Input: part model. Units: mm. Frame: model coordinates. A direction names the side the tool comes from. Round coordinates to 2 decimals unless told otherwise and drop trailing zeros. Write each loop counter-clockwise with the first axis right and the second up, starting at its lowest first coordinate (ties: lowest second). Pieces come first, ordered by that corner, then holes. Notation, with made-up numbers: (-22, 40.25) - (-9, 40.25) arc R18 ccw to (-9, 66.25) - close; hole circle Ø11 at (18.5, -10.75). An arc over 180 degrees is marked (long way). One line per item, written item: value. Start each with the question number.
Autodesk Inventor part; units mm, degrees
ref_plane "YZ Plane" through (0, 0, 0) normal (1, 0, 0) x (0, 1, 0)
ref_plane "XZ Plane" through (0, 0, 0) normal (0, 1, 0) x (-1, 0, 0)
ref_plane "XY Plane" through (0, 0, 0) normal (0, 0, 1) x (1, 0, 0)
sketch "Sketch1" plane through (0, 0, 0) normal (0, 0, 1) x (1, 0, 0)
  circle A0 centre (0, 0) radius 15
  dimension "d0" = 30
extrude "Extrusion1" add sketch "Sketch1" along normal blind 19
sketch "Sketch2" plane through (0, 0, 19) normal (0, 0, 1) x (1, 0, 0)
  circle A0 centre (0, 0) radius 3
  dimension "d3" = 6
extrude "Extrusion2" cut sketch "Sketch2" against normal blind 19
sketch "Sketch3" plane through (0, 0, 0) normal (0, 0, -1) x (-1, 0, 0)
  circle A0 centre (0, 0) radius 15
extrude "Extrusion3" add sketch "Sketch3" along normal blind 5
sketch "Sketch6" plane through (0, 0, -5) normal (0, 0, -1) x (-1, 0, 0)
  line L0 (0, -8) -> (-6.9282, -4)
  line L1 (-6.9282, -4) -> (-6.9282, 4)
  line L2 (-6.9282, 4) -> (0, 8)
  line L3 (0, 8) -> (6.9282, 4)
  line L4 (6.9282, 4) -> (6.9282, -4)
  line L5 (6.9282, -4) -> (0, -8)
  point P0 (0, 0)
  point P1 (0, 0)
  dimension "d15" = 16
extrude "Extrusion6" cut sketch "Sketch6" against normal blind 5
sketch "Sketch7" plane through (0, 0, 0) normal (1, 0, 0) x (0, 1, 0)
  circle A0 centre (0, 10) radius 1.4
  point P0 (0, 0)
  dimension "d18" = 2.8
  dimension "d19" = 10
extrude "Extrusion7" cut sketch "Sketch7" along normal through all
properties part number "FA012" material "ABS Plastic"
Q1. Pull-direction query (Y, two-part tool) for faces 3 (the flat face through (-3.1, -6.5, -5)), 4 (the cylindrical face through (8.74, -0.303, 11.367)), 5 (the flat face through (-3.416, 6.028, -2.535)); classes: pulls with the +Y half, pulls with the -Y half, needs draft (parallel to the pull), parting line crosses it, or undercut.
Q2. Cut plane B-B, the plane y = 0. Output: boundary loops of the cut face in (x, z), and give its area (3 significant figures).
Q3. Contact query for flat-ended pins moving along their axis: pin 1 Ø1.5 at (y, z) = (-10.5, 0.5) entering from +X; pin 2 Ø1.5 at (y, z) = (2, -2.5) entering from -X; pin 3 Ø1.5 at (x, z) = (9, 7.5) entering from -Y; pin 4 Ø3.5 at (x, y) = (0, 0) entering from -Z. Output: stop coordinate, or through.
Q4. Material intervals for probe 1 along Y at (x, z) = (0, 11.75); probe 2 along X at (y, z) = (6, -2.25); probe 3 along Y at (x, z) = (7.25, 10), sorted ascending. Write a range as from..to.
Q5. Cut plane C-C, the plane x = 0.5. Output: boundary loops of the cut face in (y, z), and give its area (3 significant figures).
Q6. Access query for faces 1 (the cylindrical face through (-3, 0, 10)), 2 (the flat face through (-3.513, -5.972, -2.535)). Directions: +Z, -Z, +X, -X, +Y, -Y. A direction counts if a zero-diameter tool reaches every point of the face in a straight line with its end or side. Return the directions, or none.
Q7. Cut plane D-D, the plane y = -5.5. Output: boundary loops of the cut face in (x, z).
Q8. Cut plane A-A, the plane z = -1.25. Output: boundary loops of the cut face in (x, y), and give its area (3 significant figures).
A:
1. face 3: needs draft
1. face 4: undercut
1. face 5: undercut
2. outline: (-15, -5) - (-6.93, -5) - (-6.93, 0) - (-3, 0) - (-3, 19) - (-15, 19) - close; (3, 0) - (6.93, 0) - (6.93, -5) - (15, -5) - (15, 8.6) - (3, 8.6) - close; (3, 11.4) - (15, 11.4) - (15, 19) - (3, 19) - close
2. area: 503 mm²
3. pin 1: stops at x = 11.4
3. pin 2: stops at x = -14.95
3. pin 3: stops at y = -12.53
3. pin 4: passes through
4. probe 1: y = -15..-3, 3..15
4. probe 2: x = -13.75..-3.46, 3.46..13.75
4. probe 3: y = -13.13..-1.4, 1.4..13.13
5. outline: (-14.99, -5) - (-7.71, -5) - (-7.71, 0) - (-2.96, 0) - (-2.96, 19) - (-14.99, 19) - close; (2.96, 0) - (7.71, 0) - (7.71, -5) - (14.99, -5) - (14.99, 19) - (2.96, 19) - close
5. area: 530 mm²
6. face 1: +Z, -Z
6. face 2: -Z
7. outline: (-13.96, -5) - (-4.33, -5) - (-4.33, 0) - (4.33, 0) - (4.33, -5) - (13.96, -5) - (13.96, 19) - (-13.96, 19) - close
8. outline: circle Ø30 at (0, 0); hole (-6.93, -4) - (0, -8) - (6.93, -4) - (6.93, 4) - (0, 8) - (-6.93, 4) - close
8. area: 541 mm²
